from build123d import *

# Parameters (mm, degrees)
BOSS_EXTRUDE1_DEPTH = 25


with BuildPart() as part:
    # Sketch1 → Boss-Extrude1 (new body)
    with BuildSketch(Plane.XY):
        with BuildLine():
            Line((-20, 20), (-10, 20))
            ThreePointArc((-10, 20), (-7.071067812, 12.928932188), (0, 10))
            Line((0, 10), (0, 0))
            ThreePointArc((0, 0), (-7.071067812, 2.928932188), (-10, 10))
            Line((-10, 10), (-20, 20))
        make_face()
    extrude(amount=BOSS_EXTRUDE1_DEPTH)


solid = part.part
Work out the finished part from the listing and answer in its coordinate system (mm). Give positions to 0.01 mm unless a question says otherwise; leave off trailing zeros. Write each loop counter-clockwise with the first axis right and the second up, starting at its lowest first coordinate (ties: lowest second). Pieces come first, ordered by that corner, then holes. Notation, with made-up numbers: (62.5, 50) - (66.5, 50) arc R18 cw to (66.5, 59) - close; hole circle Ø1 at (-16.75, 16.25). An arc over 180 degrees is marked (long way). One line per item, written item: value. Start each with the question number.
1. Consider probe 1 along Y at (x, z) = (-3.25, 20); probe 2 along X at (y, z) = (4.75, 4.25); probe 3 along Y at (x, z) = (-4.25, 3.5). Determine where each line is inside the solid, lowest interval first.
2. Find section A-A (z = 21.25). Write down the section's boundary in (x, y).
3. Find section C-C (y = 14). Write down the section's boundary in (x, z), then the cut area to 3 significant figures.
4. Given pin 1 (12 mm diameter, centred on x = -9, z = 7.5, fed in from -Y); pin 2 (3 mm diameter, centred on x = -7, z = 8, fed in from +Y); pin 3 (4 mm diameter, centred on x = -9, z = 17.5, fed in from -Y), each flat-ended and moving along its own axis, determine where each tip first touches the part or whether it passes through.
5. Find section B-B (x = -13). Write down the section's boundary in (y, z).
Geometry results:
1. probe 1: 0.54 to 10.54
1. probe 2: -8.51 to 0
1. probe 3: 0.95 to 10.95
2. outline: (-20, 20) - (-10, 10) arc R10 ccw to (0, 0) - (0, 10) arc R10 cw to (-10, 20) - close
3. outline: (-14, 0) - (-8, 0) - (-8, 25) - (-14, 25) - close
3. area: 150 mm2
4. pin 1: y = 0.46
4. pin 2: y = 14.73
4. pin 3: y = 2.86
5. outline: (13, 0) - (20, 0) - (20, 25) - (13, 25) - close
